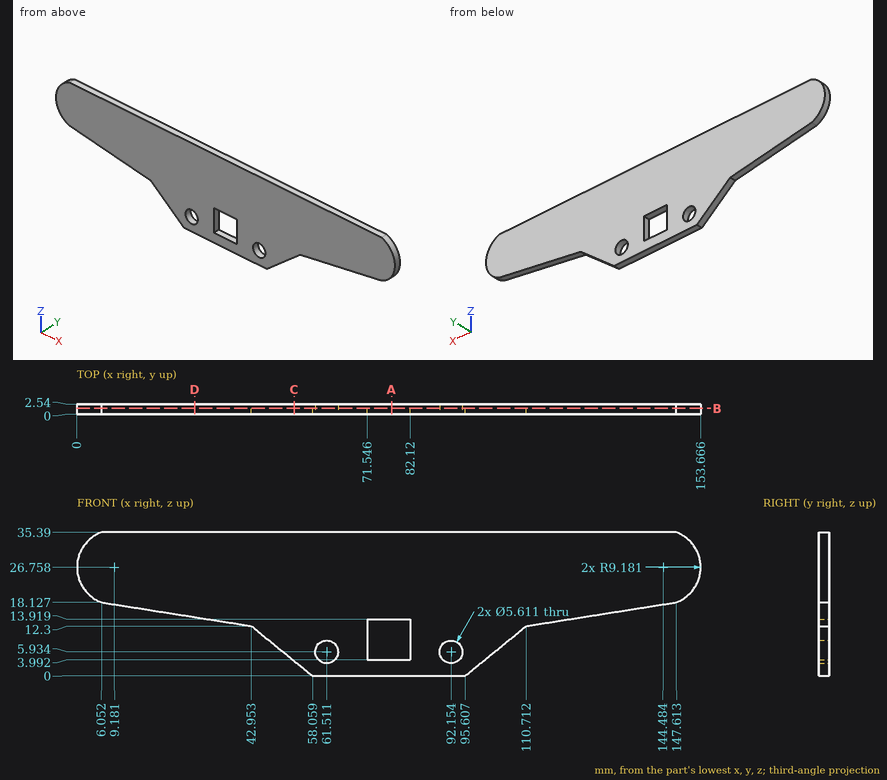
Job drawing, mm, ordinate dimensions from the low corner. One solid piece. Give positions to 0.01 mm unless a question says otherwise; leave off trailing zeros. Loops run counter-clockwise (first coordinate to the right, second up) from the corner with the lowest first, then second, coordinate; pieces in that order, holes last. Notation, with made-up numbers: M 87,42 L 94,42 A27 cw 94,72 Z; hole C 27,27.5 d1. An arc over 180 degrees is marked long. Answer in a Markdown table with one row per item. Add a question column.
Item 1: Drop flat-ended pins along their axis: P1, Ø1.5, axis at x = 127, y = 1.5, coming from the -Z side; P2, Ø0.8, axis at y = 1.5, z = 10, coming from the +X side; P3, Ø1.5, axis at y = 1.5, z = 29.5, coming from the -X side. Give the stop position or say it passes through.
Item 2: Probe probe 1 along Z at (x, y) = (61.5, 1.65); probe 2 along X at (y, z) = (0.5, 6.5) (1 decimal); probe 3 along X at (y, z) = (0.3, 26) (1 decimal). List the from-to ranges inside material, lowest first.
Item 3: Band-saw the part on D-D on x = 29. Give the cut face in (y, z).
Item 4: Band-saw the part on C-C on x = 53.5. Give the cut face in (y, z).
Item 5: Band-saw the part on B-B on y = 1.45. Give the cut face in (x, z) (1 decimal), then the cut area to 3 significant figures.
Item 6: Band-saw the part on A-A on x = 77.5. Give the cut face in (y, z).
Reply:
| question | item | result |
|---|---|---|
| 1 | P1 | stops at z = 14.75 |
| 1 | P2 | stops at x = 108.38 |
| 1 | P3 | stops at x = 0.22 |
| 2 | probe 1 | z = 0 to 3.13, 8.74 to 35.39 |
| 2 | probe 2 | x = 50.1 to 58.8, 64.3 to 71.5, 82.1 to 89.4, 94.9 to 103.6 |
| 2 | probe 3 | x = 0 to 153.6 |
| 3 | outline | M 0,14.5 L 2.54,14.5 L 2.54,35.39 L 0,35.39 Z |
| 4 | outline | M 0,3.71 L 2.54,3.71 L 2.54,35.39 L 0,35.39 Z |
| 5 | outline | M 6.1,18.1 L 43,12.3 L 58.1,0 L 95.6,0 L 110.7,12.3 L 147.6,18.1 A9.2 ccw 147.6,35.4 L 6.1,35.4 A9.2 ccw Z; hole C 61.5,5.9 d5.6; hole M 71.5,4 L 82.1,4 L 82.1,13.9 L 71.5,13.9 Z; hole C 92.2,5.9 d5.6 |
| 5 | area | 3,700 mm^2 |
| 6 | outline | M 0,0 L 2.54,0 L 2.54,3.99 L 0,3.99 Z; M 0,13.92 L 2.54,13.92 L 2.54,35.39 L 0,35.39 Z |
